```python
from build123d import *

# Parameters (mm, degrees)
F0_R        = 3
F1_DEPTH    = 10
F2_T1_DEPTH = 52.3011751173
F2_T4_ANGLE = 6.7239804363
F2_T6_ANGLE = 10.729424982
F2_T8_ANGLE = 1.7828949869


# Not quite as in the source:
# - a fillet or chamfer that OpenCascade refuses, or shapes differently, is made with other operations: its cross-section is extruded or revolved along the edge and cut away or added


with BuildPart() as f1:
    # F0 (on Front) → F1 (new body)
    with BuildSketch(Plane.XZ):
        with BuildLine():
            ThreePointArc((16.7161625637, 9.1005522793), (15.1603559483, 9.0884488757), (13.604925944, 9.0521415948))
            ThreePointArc((13.604925944, 9.0521415948), (-24.5259537531, 6.9533029462), (-62.5132279063, 3.0371680453))
            ThreePointArc((-62.5132279063, 3.0371680453), (-63.4446975244, -7.2627028514), (-59.2295458713, -16.7066147888))
            ThreePointArc((-59.2295458713, -16.7066147888), (-3.9332598443, -11.7153648591), (51.5779973344, -10.6703047235))
            ThreePointArc((51.5779973344, -10.6703047235), (52.7884384629, -0.7810693697), (51.517337681, 9.1005522793))
            Line((51.517337681, 9.1005522793), (16.7161625637, 9.1005522793))
        make_face()
        with Locations((-33.4603461426, -3.8443253384)):
            Circle(F0_R, mode=Mode.SUBTRACT)
        with Locations((22.7880547631, -0.7167291473)):
            Circle(F0_R, mode=Mode.SUBTRACT)
    extrude(amount=F1_DEPTH)

    # F2: fillet of radius 7 on 4 edges, made by hand

    # F2_s2 → F2_t1 (cut)
    with BuildSketch(Plane.YZ.offset(16.7161625637)):
        with BuildLine():
            ThreePointArc((-3, 9.1005522793), (-7.9497474683, 7.0502997476), (-10, 2.1005522793))
            Line((-10, 2.1005522793), (-10, 9.1005522793))
            Line((-10, 9.1005522793), (-3, 9.1005522793))
        make_face()
    extrude(amount=F2_T1_DEPTH, mode=Mode.SUBTRACT)

    # F2_s3 → F2_t4 (revolve, cut)
    with BuildSketch(Plane(origin=(13.8732538603, 0, 0.4318388106), x_dir=(0, 1, 0), z_dir=(0.9995158932, 0, 0.0311123662))):
        with BuildLine():
            ThreePointArc((-3, 8.624477953), (-7.9497474683, 6.5742254213), (-10, 1.624477953))
            Line((-10, 1.624477953), (-10, 8.624477953))
            Line((-10, 8.624477953), (-3, 8.624477953))
        make_face()
    revolve(axis=Axis((38.4948189015, -10, -790.5605729296), (0, -1, 0)), revolution_arc=F2_T4_ANGLE, mode=Mode.SUBTRACT)

    # F2_s5 → F2_t6 (revolve, cut)
    with BuildSketch(Plane(origin=(-77.6853434409, 0, -11.5863862591), x_dir=(0, 1, 0), z_dir=(-0.9890600521, 0, -0.1475134342))):
        with BuildLine():
            ThreePointArc((-3, 7.5903844134), (-7.9497474683, 5.5401318817), (-10, 0.5903844134))
            Line((-10, 0.5903844134), (-10, 7.5903844134))
            Line((-10, 7.5903844134), (-3, 7.5903844134))
        make_face()
    revolve(axis=Axis((38.4948189015, -10, -790.5605729293), (0, 1, 0)), revolution_arc=F2_T6_ANGLE, mode=Mode.SUBTRACT)

    # F2_s7 → F2_t8 (revolve, cut)
    with BuildSketch(Plane.YZ.offset(16.7161625637)):
        with BuildLine():
            ThreePointArc((-3, 9.1005522793), (-7.9497474683, 7.0502997476), (-10, 2.1005522793))
            Line((-10, 2.1005522793), (-10, 9.1005522793))
            Line((-10, 9.1005522793), (-3, 9.1005522793))
        make_face()
    revolve(axis=Axis((16.7161625637, -10, -90.8994477206), (0, -1, 0)), revolution_arc=F2_T8_ANGLE, mode=Mode.SUBTRACT)


solid = f1.part
```
Work out the finished part from the listing and answer in its coordinate system (mm). A direction names the side the tool comes from. Coordinates: 2 decimals unless noted, no trailing zeros. Loops run counter-clockwise (first coordinate to the right, second up) from the corner with the lowest first, then second, coordinate; pieces in that order, holes last.
1) Consider probe 1 along X at (y, z) = (-3.75, -0.75); probe 2 along Z at (x, y) = (27, -1.75); probe 3 along X at (y, z) = (-5.25, -6.25). Determine where each line is inside the solid, lowest interval first.
Results:
probe 1: x = -63.48 to 19.79, 25.79 to 52.79
probe 2: z = -10.65 to 9.1
probe 3: x = -63.59 to -35.25, -31.67 to 52.43
2) For a pull along X with two mould halves and no side action, classify faces 1 (the cylindrical face through (-36.457, -4.93, -3.712)), 2 (the flat face through (-6, 0, -4)), 3 (the cylindrical face through (52.79, -4.93, -0.92)), 4 (the cylindrical face through (25.559, -4.93, -1.866)) as +X half, -X half, draft (parallel to the pull), parting line (faces both ways), or undercut.
Results:
face 1: undercut
face 2: draft
face 3: +X half
face 4: undercut
3) Section A-A (y = -5.5) is taken. Give the vertices of the cut face in (x, z).
Results:
outline: (-62.68, 2.55) arc R20.5 ccw to (-59.56, -16.28) arc R780.46 cw to (51.69, -10.21) arc R40 ccw to (51.63, 8.64) - (16.72, 8.64) arc R99.54 ccw to (13.62, 8.59) arc R799.54 ccw to start; hole circle Ø6 at (-33.46, -3.84); hole circle Ø6 at (22.79, -0.72)
4) Flat-ended cylindrical pins translate along their axes: pin 1 (10 mm diameter, centred on x = 5.5, z = -13, fed in from -Y); pin 2 (1.5 mm diameter, centred on y = -9, z = -14, fed in from -X); pin 3 (1 mm diameter, centred on x = -45.5, y = -8.5, fed in from +Z). Find the tip coordinate at first contact, or state that the pin passes through.
Results:
pin 1: stops at y = -8.92
pin 2: stops at x = -61.47
pin 3: stops at z = 2.91
5) For faces 5 (the cylindrical face through (34, -8, 7)), 6 (the cylindrical face through (-4.71, -1.48, -11.76)), determine the directions among +Z, -Z, +X, -X, +Y, -Y from which every point of the face is accessible in a straight line to the end or side of a thin tool.
Results:
face 5: +Z, +X, -X, -Y
face 6: -Z, +Y, -Y
